from build123d import *

# Parameters (mm, degrees)
SKETCH1_R                = 16.25
SKETCH1_W                = 121
SKETCH1_H                = 110
BOSS_EXTRUDE1_DEPTH      = 11
SKETCH1_5_W              = 121
SKETCH1_5_H              = 110
SKETCH1_5_W_2            = 101
SKETCH1_5_H_2            = 90
BOSS_EXTRUDE2_DEPTH      = 12.5
SKETCH1_7_W              = 101
SKETCH1_7_H              = 90
SKETCH1_7_W_2            = 98
SKETCH1_7_H_2            = 87
BOSS_EXTRUDE3_DEPTH      = 10
SKETCH1_8_W              = 98
SKETCH1_8_H              = 87
SKETCH1_8_W_2            = 92
SKETCH1_8_H_2            = 81
BOSS_EXTRUDE4_DEPTH      = 9
SKETCH1_9_R              = 16.25
SKETCH1_9_R_2            = 10.25
BOSS_EXTRUDE5_DEPTH      = 5.5
OLES_RUNDING_R           = 11.65
FILLET7_R                = 1
FILLET8_R                = 4
FILLET9_R                = 5.5
M3_TAPPED_HOLE1_D        = 2.5
M4_TAPPED_HOLE2_D        = 3.3
M4_TAPPED_HOLE2_DEPTH    = 10.1
M4_TAPPED_HOLE2_TIP      = 0.991420021
FILLET11_R               = 5
M3_TAPPED_HOLE3_D        = 2.5
M3_TAPPED_HOLE3_DEPTH    = 9.5
M3_TAPPED_HOLE3_TIP      = 0.751075774
BOSS_EXTRUDE6_START      = 5
BOSS_EXTRUDE6_DEPTH      = 5
FILLET12_R               = 25
FILLET13_R               = 22
FILLET14_R               = 21.3
M6_CLEARANCE_HOLE4_D     = 6.6
CUT_EXTRUDE1_DEPTH       = 158.634775668
CUT_EXTRUDE1_DEPTH_BACK  = 158.634775668
FILLET15_START           = 11
FILLET15_DEPTH           = 5
BOSS_EXTRUDE7_DEPTH      = 5
BOSS_EXTRUDE7_DEPTH_BACK = 11
CUT_EXTRUDE2_DEPTH       = 164.158772366
CUT_EXTRUDE2_DEPTH_BACK  = 164.158772366
SKETCH26_3_R             = 3.25
FILLET16_R               = 3
JENS_S_RUNDING_R         = 35


with BuildPart() as part:
    # Sketch1 → Boss-Extrude1 (new body)
    with BuildSketch(Plane.XY):
        Polygon((-121.65, -86), (121.65, -86), (131.65, -86), (131.65, -55), (131.65, -30), (121.65, -30), (121.65, 30), (131.65, 30), (131.65, 55), (131.65, 70), (131.65, 86), (121.65, 86), (-121.65, 86), (-126.65, 86), (-126.65, -86), align=None)
        with Locations((-100.35, 0)):
            Circle(SKETCH1_R, mode=Mode.SUBTRACT)
        with Locations((37.25, 0)):
            Rectangle(SKETCH1_W, SKETCH1_H, mode=Mode.SUBTRACT)
    extrude(amount=BOSS_EXTRUDE1_DEPTH)

    # Sketch1<5> → Boss-Extrude2 (add)
    with BuildSketch(Plane.XY):
        with Locations((37.25, 0)):
            Rectangle(SKETCH1_5_W, SKETCH1_5_H)
        with Locations((37.25, 0)):
            Rectangle(SKETCH1_5_W_2, SKETCH1_5_H_2, mode=Mode.SUBTRACT)
    extrude(amount=BOSS_EXTRUDE2_DEPTH)

    # Sketch1<7> → Boss-Extrude3 (add)
    with BuildSketch(Plane.XY):
        with Locations((37.25, 0)):
            Rectangle(SKETCH1_7_W, SKETCH1_7_H)
        with Locations((37.25, 0)):
            Rectangle(SKETCH1_7_W_2, SKETCH1_7_H_2, mode=Mode.SUBTRACT)
    extrude(amount=BOSS_EXTRUDE3_DEPTH)

    # Sketch1<8> → Boss-Extrude4 (add)
    with BuildSketch(Plane.XY):
        with Locations((37.25, 0)):
            Rectangle(SKETCH1_8_W, SKETCH1_8_H)
        with Locations((37.25, 0)):
            Rectangle(SKETCH1_8_W_2, SKETCH1_8_H_2, mode=Mode.SUBTRACT)
    extrude(amount=BOSS_EXTRUDE4_DEPTH)

    # Sketch1<9> → Boss-Extrude5 (add)
    with BuildSketch(Plane.XY):
        with Locations((-100.35, 0)):
            Circle(SKETCH1_9_R)
        with Locations((-100.35, 0)):
            Circle(SKETCH1_9_R_2, mode=Mode.SUBTRACT)
    extrude(amount=BOSS_EXTRUDE5_DEPTH)

    # oles runding
    oles_runding_edges = [part.edges().sort_by_distance(p)[0] for p in [
        (-23.25, 55, 11.75),
        (-23.25, -55, 11.75),
        (97.75, -55, 11.75),
        (97.75, 55, 11.75),
    ]]
    fillet(oles_runding_edges, radius=OLES_RUNDING_R)

    # Fillet7
    fillet7_edges = [part.edges().sort_by_distance(p)[0] for p in [
        (83.25, -40.5, 4.5),
        (-8.75, -40.5, 4.5),
        (-8.75, 40.5, 4.5),
        (83.25, 40.5, 4.5),
    ]]
    fillet(fillet7_edges, radius=FILLET7_R)

    # Fillet8
    fillet8_edges = [part.edges().sort_by_distance(p)[0] for p in [
        (86.25, -43.5, 9.5),
        (-11.75, -43.5, 9.5),
        (-11.75, 43.5, 9.5),
        (86.25, 43.5, 9.5),
    ]]
    fillet(fillet8_edges, radius=FILLET8_R)

    # Fillet9
    fillet9_edges = [part.edges().sort_by_distance(p)[0] for p in [
        (87.75, -45, 11.25),
        (-13.25, -45, 11.25),
        (-13.25, 45, 11.25),
        (87.75, 45, 11.25),
    ]]
    fillet(fillet9_edges, radius=FILLET9_R)

    # M3 Tapped Hole1 (through all)
    with Locations(Plane.XY.offset(5.5)):
        with Locations((-89.091669751, 6.5), (-100.35, -13), (-111.608330249, 6.5)):
            Hole(M3_TAPPED_HOLE1_D / 2)

    # M4 Tapped Hole2
    with Locations(Plane(origin=(121.65, 0, 0), x_dir=(0, 0, -1), z_dir=(1, 0, 0))):
        with Locations((-6, 17), (-6, -17)):
            Hole(M4_TAPPED_HOLE2_D / 2, depth=M4_TAPPED_HOLE2_DEPTH)
            with Locations((0, 0, -(M4_TAPPED_HOLE2_DEPTH + M4_TAPPED_HOLE2_TIP / 2))):  # 118° drill point
                Cone(0, M4_TAPPED_HOLE2_D / 2, M4_TAPPED_HOLE2_TIP, mode=Mode.SUBTRACT)

    # Fillet11
    fillet11_edges = [part.edges().sort_by_distance(p)[0] for p in [
        (121.65, -30, 5.5),
        (121.65, 30, 5.5),
    ]]
    fillet(fillet11_edges, radius=FILLET11_R)
    fillet11_2_edges = [part.edges().sort_by_distance(p)[0] for p in [
        (131.65, -30, 5.5),
        (131.65, 30, 5.5),
    ]]
    fillet(fillet11_2_edges, radius=FILLET11_R - 0.0001)  # a hair under: the kernel refuses the full size

    # M3 Tapped Hole3
    with Locations(Plane.XY.offset(12.5)):
        with Locations((-15.738440649, -47.488440649), (-15.738440649, 47.488440649), (90.238440649, 47.488440649), (90.238440649, -47.488440649)):
            Hole(M3_TAPPED_HOLE3_D / 2, depth=M3_TAPPED_HOLE3_DEPTH)
            with Locations((0, 0, -(M3_TAPPED_HOLE3_DEPTH + M3_TAPPED_HOLE3_TIP / 2))):  # 118° drill point
                Cone(0, M3_TAPPED_HOLE3_D / 2, M3_TAPPED_HOLE3_TIP, mode=Mode.SUBTRACT)

    # Sketch20 → Boss-Extrude6 (add)
    with BuildSketch(Plane.XY.offset(11).offset(BOSS_EXTRUDE6_START)):
        with BuildLine():
            Line((121.65, -25), (121.65, -76))
            Line((121.65, -76), (-78.35, -76))
            Line((-78.35, -76), (-78.35, -21.3))
            Line((-78.35, -21.3), (-121.65, -21.3))
            Line((-121.65, -21.3), (-121.65, 21.3))
            Line((-121.65, 21.3), (-78.35, 21.3))
            Line((-78.35, 21.3), (-78.35, 76))
            Line((-78.35, 76), (31.535138546, 76))
            Line((31.535138546, 76), (61.535138546, 76))
            Line((61.535138546, 76), (121.65, 76))
            Line((121.65, 76), (121.65, 25))
            ThreePointArc((121.65, 25), (123.114466094, 28.535533906), (126.65, 30))
            ThreePointArc((126.65, 30), (130.185533906, 31.464466094), (131.65, 35))
            Line((131.65, 35), (131.65, 86))
            Line((131.65, 86), (-126.65, 86))
            Line((-126.65, 86), (-126.65, -86))
            Line((-126.65, -86), (131.65, -86))
            Line((131.65, -86), (131.65, -35))
            ThreePointArc((131.65, -35), (130.185533906, -31.464466094), (126.65, -30))
            ThreePointArc((126.65, -30), (123.114466094, -28.535533906), (121.65, -25))
        make_face()
    extrude(amount=-BOSS_EXTRUDE6_DEPTH)

    # Fillet12
    fillet12_edges = [part.edges().sort_by_distance(p)[0] for p in [
        (-126.65, -86, 8),
        (-126.65, 86, 8),
        (121.65, -76, 13.5),
        (-78.35, -76, 13.5),
        (-78.35, 76, 13.5),
        (121.65, 76, 13.5),
    ]]
    fillet(fillet12_edges, radius=FILLET12_R)

    # Fillet13
    fillet13_edges = [part.edges().sort_by_distance(p)[0] for p in [
        (-78.35, -21.3, 13.5),
        (-78.35, 21.3, 13.5),
    ]]
    fillet(fillet13_edges, radius=FILLET13_R)

    # Fillet14
    fillet14_edges = [part.edges().sort_by_distance(p)[0] for p in [
        (-121.65, -21.3, 13.5),
        (-121.65, 21.3, 13.5),
    ]]
    fillet(fillet14_edges, radius=FILLET14_R - 0.0001)  # a hair under: the kernel refuses the full size

    # M6 Clearance Hole4 (through all)
    with Locations(Plane.XY.offset(16)):
        with Locations((-99.95, 37.5), (-99.95, -37.5)):
            Hole(M6_CLEARANCE_HOLE4_D / 2)

    # Sketch25 → Cut-Extrude1 (cut, two sides: drawn at the far end of the back side and taken through both)
    with BuildSketch(Plane.XY.offset(11).offset(-CUT_EXTRUDE1_DEPTH_BACK)):
        with BuildLine():
            Line((52.25, 86), (22.25, 86))
            ThreePointArc((22.25, 86), (25.178932188, 78.928932188), (32.25, 76))
            Line((32.25, 76), (42.25, 76))
            ThreePointArc((42.25, 76), (49.321067812, 78.928932188), (52.25, 86))
        make_face()
    extrude(amount=CUT_EXTRUDE1_DEPTH + CUT_EXTRUDE1_DEPTH_BACK, mode=Mode.SUBTRACT)

    # Fillet15: read off the stored shape, not the designer's step
    # Fillet15 outline → Fillet15 (cut)
    with BuildSketch(Plane.XY.offset(FILLET15_START)):
        with BuildLine():
            Line((121.65, -25), (121.65, -29.472135955))
            ThreePointArc((121.65, -29.472135955), (122.24175171, -28.559265026), (123.316666667, -28.726779962))
            ThreePointArc((123.316666667, -28.726779962), (122.085645354, -27.041241452), (121.65, -25))
        make_face()
        with BuildLine():
            ThreePointArc((123.316666667, 28.726779962), (122.24175171, 28.559265026), (121.65, 29.472135955))
            Line((121.65, 29.472135955), (121.65, 25))
            ThreePointArc((121.65, 25), (122.085645354, 27.041241452), (123.316666667, 28.726779962))
        make_face()
        with BuildLine():
            ThreePointArc((48.57455532, 76), (47.621092731, 76.698488655), (47.999595746, 77.818181818))
            ThreePointArc((47.999595746, 77.818181818), (45.265113446, 76.465374107), (42.25, 76))
            Line((42.25, 76), (48.57455532, 76))
        make_face()
        with BuildLine():
            ThreePointArc((26.500404254, 77.818181818), (26.878907269, 76.698488655), (25.92544468, 76))
            Line((25.92544468, 76), (32.25, 76))
            ThreePointArc((32.25, 76), (29.234886554, 76.465374107), (26.500404254, 77.818181818))
        make_face()
    extrude(amount=FILLET15_DEPTH, mode=Mode.SUBTRACT)

    # Sketch26 → Boss-Extrude7 (add, two sides: drawn at the far end of the back side and taken through both)
    with BuildSketch(Plane.XY.offset(11).offset(-BOSS_EXTRUDE7_DEPTH_BACK)):
        with BuildLine():
            Line((72.166859351, -86), (66.8, -86))
            Line((66.8, -86), (66.8, -95.75))
            Line((66.8, -95.75), (83.3, -95.75))
            Line((83.3, -95.75), (83.3, -86))
            Line((83.3, -86), (77.933140649, -86))
            ThreePointArc((77.933140649, -86), (78.206953207, -86.727894796), (78.3, -87.5))
            ThreePointArc((78.3, -87.5), (74.277894796, -90.656953207), (72.166859351, -86))
        make_face()
        with BuildLine():
            Line((66.8, 95.75), (66.8, 86))
            Line((66.8, 86), (72.166859351, 86))
            ThreePointArc((72.166859351, 86), (74.277894796, 90.656953207), (78.3, 87.5))
            ThreePointArc((78.3, 87.5), (78.206953207, 86.727894796), (77.933140649, 86))
            Line((77.933140649, 86), (83.3, 86))
            Line((83.3, 86), (83.3, 95.75))
            Line((83.3, 95.75), (66.8, 95.75))
        make_face()
    extrude(amount=BOSS_EXTRUDE7_DEPTH + BOSS_EXTRUDE7_DEPTH_BACK)

    # Sketch26<3> → Cut-Extrude2 (cut, two sides: drawn at the far end of the back side and taken through both)
    with BuildSketch(Plane.XY.offset(11).offset(-CUT_EXTRUDE2_DEPTH_BACK)):
        with Locations((75.05, -87.5)):
            Circle(SKETCH26_3_R)
        with Locations((75.05, 87.5)):
            Circle(SKETCH26_3_R)
    extrude(amount=CUT_EXTRUDE2_DEPTH + CUT_EXTRUDE2_DEPTH_BACK, mode=Mode.SUBTRACT)

    # Fillet16
    fillet16_edges = [part.edges().sort_by_distance(p)[0] for p in [
        (83.3, -86, 8),
        (83.3, -95.75, 8),
        (66.8, -95.75, 8),
        (66.8, -86, 8),
        (66.8, 86, 8),
        (66.8, 95.75, 8),
        (83.3, 95.75, 8),
        (83.3, 86, 8),
    ]]
    fillet(fillet16_edges, radius=FILLET16_R)

    # Jens's runding
    jens_s_runding_edges = [part.edges().sort_by_distance(p)[0] for p in [
        (131.65, -86, 8),
        (131.65, 86, 8),
    ]]
    fillet(jens_s_runding_edges, radius=JENS_S_RUNDING_R)


solid = part.part
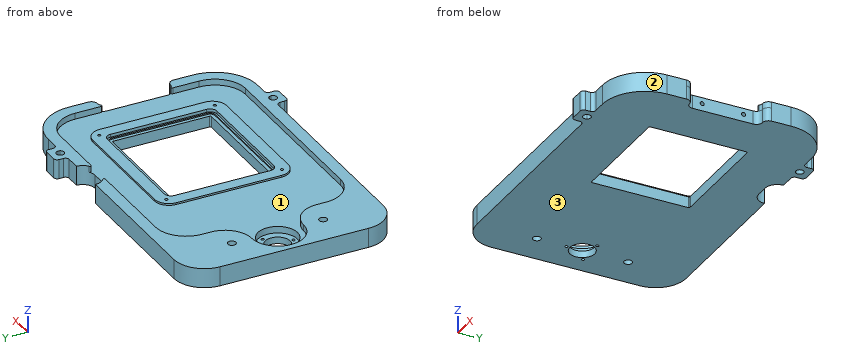
Build history of the part. All positions in model axes, mm. Face numbers are marked on the shaded views. Round coordinates to 2 decimals unless told otherwise and drop trailing zeros. Write each loop counter-clockwise with the first axis right and the second up, starting at its lowest first coordinate (ties: lowest second). Pieces come first, ordered by that corner, then holes. Notation, with made-up numbers: (-31.75, 54) -> (-16.75, 54) arc R11 cw to (-16.75, 60) -> close; hole circle Ø1 at (83, 86). An arc over 180 degrees is marked (long way). Write item = value, one per line.
(1) Band-saw the part on C-C (y = -69). Give the cut face in (x, z).
Answer:
outline = (-125.34, 0) -> (126.67, 0) -> (126.67, 16) -> (114, 16) -> (114, 11) -> (-70.7, 11) -> (-70.7, 16) -> (-125.34, 16) -> close
(2) Probe L1, parallel to Y at x = 96, z = 13; L2, parallel to Y at x = 26.5, z = 6.5; L3, parallel to Z at x = 119, y = -17. List the from-to ranges inside material, lowest first.
Answer:
L1 = -86 to -76, 76 to 86
L2 = -86 to -40.5, 40.5 to 77.82
L3 = 0 to 4.35, 7.65 to 11
(3) Two-plate mould, pull along Y, no slides. Class the marked faces 1, 2 and 3: pulls with the +Y half, pulls with the -Y half, needs draft (parallel to the pull), parting line crosses it, or undercut.
Answer:
face_1 = undercut
face_2 = pulls with the -Y half
face_3 = needs draft
(4) Flat gauge pins, fed straight in: pin 1 (2 mm diameter, centred on x = 84.5, y = -28, fed in from +Z); pin 2 (2 mm diameter, centred on y = 70, z = 8.5, fed in from -X); pin 3 (4 mm diameter, centred on x = -68, z = 10.5, fed in from -Y); pin 4 (16.5 mm diameter, centred on x = -100.35, y = 0, fed in from -Z). Where does each tip first touch, or does it go through?
Answer:
pin_1 = 9
pin_2 = -125.34
pin_3 = -86
pin_4 = through
(5) Band-saw the part on A-A (x = 75.05). State how many separate pieces and enclosed holes the cut face has, then the cut area to 3 significant figures.
Answer:
separate_pieces = 4
enclosed_holes = 0
area = 1,220 mm2
(6) Band-saw the part on B-B (x = -28.5). Give the cut face in (y, z).
Answer:
outline = (-86, 0) -> (86, 0) -> (86, 16) -> (76, 16) -> (76, 11) -> (-76, 11) -> (-76, 16) -> (-86, 16) -> close
